Here's how the part is built. I have some questions about the finished solid (model axes, mm). A direction names the side the tool comes from. Give positions to 0.01 mm unless a question says otherwise; leave off trailing zeros. Write each loop counter-clockwise with the first axis right and the second up, starting at its lowest first coordinate (ties: lowest second). Pieces come first, ordered by that corner, then holes. Notation, with made-up numbers: (73, 18) - (86, 18) arc R26 cw to (86, 35) - close; hole circle Ø11 at (15, -18.75). An arc over 180 degrees is marked (long way). One line per item, written item: value. Start each with the question number.
1) I'm going to push flat-ended pins straight in: P1, Ø1.5, axis at x = 11.5, y = 8.5, coming from the +Z side; P2, Ø3, axis at x = 1.5, z = 9.5, coming from the +Y side; P3, Ø6, axis at y = -5, z = 7.5, coming from the +X side; P4, Ø12, axis at x = 0, y = 0, coming from the +Z side. Where does each tip first touch, or does it pass through?
2) On a 3-axis mill with a long thin cutter (end or side, diameter ignored), from which of +Z, -Z, +X, -X, +Y, -Y can I reach the whole of each face in a straight line? I mean faces 5 (the flat face through (-1.5, -9, 3)), 6 (the flat face through (-2.9, 7.1, 12)). Say none if no direction works.
3) Imagine slicing it at B-B on x = 0. Write out the boundary of the cut face in (y, z), plus the area to 3 significant figures.
4) We'd pull the mould along X, two halves only. Please class faces 1 (the cylindrical face through (0.309, 7.494, 5.916)), 2 (the flat face through (1.5, -9, 3)), 3 (the cylindrical face through (0.4, 9.49, 6.93)), 4 (the flat face through (8, -7, 2)): +X half, -X half, draft (parallel to the pull), parting line (faces both ways), or undercut.
5) Imagine slicing it at D-D on z = 11. Write out the boundary of the cut face in (x, y).
6) Imagine slicing it at A-A on y = 0. Write out the boundary of the cut face in (x, z).
7) Please list where these lines run through material, in increasing order: L1, parallel to X at y = 0, z = 5.75; L2, parallel to Y at x = 0, z = 3.5; L3, parallel to Z at x = 10, y = 13. Write a range as [from, to].
8) Imagine slicing it at C-C on x = -7. Write out the boundary of the cut face in (y, z), plus the area to 3 significant figures.
from build123d import *

# Parameters (mm, degrees)
F0_R     = 17.5
F0_R_2   = 7.5
F1_DEPTH = 2
F2_R     = 9.5
F2_R_2   = 7.5
F3_DEPTH = 10
F4_W     = 3
F4_H     = 10.151531
F5_DEPTH = 12.001


with BuildPart() as f1:
    # F0 (on Top) → F1 (new body)
    with BuildSketch(Plane.XY):
        Circle(F0_R)
        Circle(F0_R_2, mode=Mode.SUBTRACT)
    extrude(amount=F1_DEPTH)

    # F2 (on face) → F3 (join)
    with BuildSketch(Plane.XY.offset(2)):
        Circle(F2_R)
        Circle(F2_R_2, mode=Mode.SUBTRACT)
    extrude(amount=F3_DEPTH)

    # F4 (on Top) → F5 (cut, through all)
    with BuildSketch(Plane.XY):
        with Locations((0, -12.424235)):
            Rectangle(F4_W, F4_H)
    extrude(amount=F5_DEPTH, mode=Mode.SUBTRACT)


solid = f1.part
Numbers:
1. P1: z = 2
1. P2: y = 9.5
1. P3: x = 9.29
1. P4: through
2. face 5: +Z, -Z, -Y
2. face 6: +Z, +X, -X, +Y, -Y
3. outline: (7.5, 0) - (17.5, 0) - (17.5, 2) - (9.5, 2) - (9.5, 12) - (7.5, 12) - close
3. area: 40.0 mm^2
4. face 1: undercut
4. face 2: undercut
4. face 3: parting line
4. face 4: draft
5. outline: (-1.5, -9.38) - (-1.5, -7.35) arc R7.5 cw (long way) to (1.5, -7.35) - (1.5, -9.38) arc R9.5 ccw (long way) to start
6. outline: (-17.5, 0) - (-7.5, 0) - (-7.5, 12) - (-9.5, 12) - (-9.5, 2) - (-17.5, 2) - close; (7.5, 0) - (17.5, 0) - (17.5, 2) - (9.5, 2) - (9.5, 12) - (7.5, 12) - close
7. L1: [-9.5, -7.5], [7.5, 9.5]
7. L2: [7.5, 9.5]
7. L3: [0, 2]
8. outline: (-16.04, 0) - (-2.69, 0) - (-2.69, 12) - (-6.42, 12) - (-6.42, 2) - (-16.04, 2) - close; (2.69, 0) - (16.04, 0) - (16.04, 2) - (6.42, 2) - (6.42, 12) - (2.69, 12) - close
8. area: 128 mm^2
